For this review, take the finished solid that the model builds, in its own axes (mm). A direction names the side the tool comes from. Coordinates: 2 decimals unless noted, no trailing zeros. Loops run counter-clockwise (first coordinate to the right, second up) from the corner with the lowest first, then second, coordinate; pieces in that order, holes last.
1. Machinability: for faces 5 (the face through (0, -2, -76)), 6 (the face through (-24.577, 1.657, -55.458)), 7 (the face through (-74, -2, 10)), 8 (the face through (1.156, 0.908, -76.264)), 9 (the face through (8.684, -1.972, 16.654)), which of the approach directions +Z, -Z, +X, -X, +Y, -Y give a long, thin tool a straight path to every point of the face, cutting with its end or side? Answer none if there is none.
2. Take a section at B-B, the plane z = -50. State the section outline as (x, y) points, then the cut area to 3 significant figures.
3. Clearance check with flat-ended pins moving along their axes: P1, Ø2.5, axis at x = -8.75, z = -15.16, coming from the +Y side; P2, Ø5, axis at x = -8.75, z = 15.16, coming from the +Y side; P3, Ø3, axis at x = -43.5, z = -1.5, coming from the +Y side; P4, Ø8, axis at y = 5.5, z = -23.5, coming from the +X side. State where each tip first meets the part, or that it passes through.
4. Mouldability with a two-part tool opening along Y and no side actions: class faces 1 (the face through (76.066, 0.908, -3.422)), 2 (the face through (-1, -2, 26)), 3 (the face through (1, -4, -13)), 4 (the face through (27, 14.523, 18)) as pulls with the +Y half, pulls with the -Y half, needs draft (parallel to the pull), parting line crosses it, or undercut.
5. Take a section at A-A, the plane y = 9.5. State the section outline as (x, z) points, then the cut area to 3 significant figures.
6. To check wall thickness, follow probe 1 along X at (y, z) = (-1.25, -16); probe 2 along Z at (x, y) = (-46, 8.25); probe 3 along Z at (x, y) = (6, 10.75). State the ranges of each line that lie inside material, in increasing order.
```python
from build123d import *

# Parameters (mm, degrees)
SKETCH_1_R          = 26
EXTRUDE_1_DEPTH     = 1
EXTRUDE_1_2_DEPTH   = 1
EXTRUDE_1_3_DEPTH   = 1
EXTRUDE_START       = 4
SKETCH_2_R          = 10
EXTRUDE_2_DEPTH     = 4
SKETCH_3_R          = 1.5
CUT_EXTRUDE_1_DEPTH = 4


with BuildPart() as part:
    # Sketch 1 → Extrude 1 (new body)
    with BuildSketch(Plane(origin=(0, 0, 0), x_dir=(1, 0, 0), z_dir=(0, 1, 0))):
        with Locations(Location((0, 50, 0), (0, 0, 270))):
            Circle(SKETCH_1_R)
    extrude(amount=EXTRUDE_1_DEPTH)



with BuildPart() as body_2:
    # Sketch 1 → Extrude 1 2 (new body)
    with BuildSketch(Plane(origin=(0, 0, 0), x_dir=(1, 0, 0), z_dir=(0, 1, 0))):
        with Locations(Location((50, 0, 0), (0, 0, 270))):
            Circle(SKETCH_1_R)
    extrude(amount=EXTRUDE_1_2_DEPTH)


with BuildPart() as body_3:
    # Sketch 1 → Extrude 1 3 (new body)
    with BuildSketch(Plane(origin=(0, 0, 0), x_dir=(1, 0, 0), z_dir=(0, 1, 0))):
        with Locations(Location((-50, 0, 0), (0, 0, 270))):
            Circle(SKETCH_1_R)
    extrude(amount=EXTRUDE_1_3_DEPTH)


with BuildPart() as part_1:
    add(part.part)

    add(body_2.part)  # Extrude 2 merges body 2

    add(body_3.part)  # Extrude 2 merges body 3
    # Sketch 2 → Extrude 2 (add)
    with BuildSketch(Plane.XZ.offset(EXTRUDE_START)):
        with BuildLine():
            Line((-50, 26), (50, 26))
            ThreePointArc((50, 26), (74.020867845, 9.949769241), (68.384776311, -18.384776311))
            Line((68.384776311, -18.384776311), (18.384776311, -68.384776311))
            ThreePointArc((18.384776311, -68.384776311), (0, -76), (-18.384776311, -68.384776311))
            Line((-18.384776311, -68.384776311), (-68.384776311, -18.384776311))
            ThreePointArc((-68.384776311, -18.384776311), (-74.020867845, 9.949769241), (-50, 26))
        make_face()
        with Locations(Location((0, 0, 0), (0, 0, 270))):
            Circle(SKETCH_2_R, mode=Mode.SUBTRACT)
    extrude(amount=-EXTRUDE_2_DEPTH)

    # Sketch 3 → Cut-Extrude 1 (cut)
    with BuildSketch(Plane(origin=(0, 0, 0), x_dir=(1, 0, 0), z_dir=(0, 1, 0))):
        with Locations(Location((8.75, 15.155444566, 0), (0, 0, 270))):
            Circle(SKETCH_3_R)
        with Locations(Location((17.5, 0, 0), (0, 0, 270))):
            Circle(SKETCH_3_R)
        with Locations(Location((-17.5, 0, 0), (0, 0, 90))):
            Circle(SKETCH_3_R)
        with Locations(Location((-8.75, 15.155444566, 0), (0, 0, 90))):
            Circle(SKETCH_3_R)
        with Locations(Location((-8.75, -15.155444566, 0), (0, 0, 270))):
            Circle(SKETCH_3_R)
        with Locations(Location((8.75, -15.155444566, 0), (0, 0, 90))):
            Circle(SKETCH_3_R)
    extrude(amount=-CUT_EXTRUDE_1_DEPTH, mode=Mode.SUBTRACT)

    # Sketch 4 → Revolve 1 (revolve)
    with BuildSketch(Plane(origin=(0, 0, 0), x_dir=(0, 0, -1), z_dir=(1, 0, 0)), mode=Mode.PRIVATE) as revolve_1_sk:
        Polygon((80.623466631, 14.522961568), (78.623466631, 14.522961568), (75, 1), (76, 1), (76, 0), align=None)
    revolve(revolve_1_sk.sketch.rotate(Axis((0, 1, -50), (0, 1, 0)), 180), axis=Axis((0, 1, -50), (0, 1, 0)))

    # Sketch 6 → Revolve 2 (revolve)
    with BuildSketch(Plane.XY, mode=Mode.PRIVATE) as revolve_2_sk:
        Polygon((-75, 1), (-78.623466631, 14.522961568), (-80.623466631, 14.522961568), (-76, 0), (-76, 1), align=None)
    revolve(revolve_2_sk.sketch.rotate(Axis((-50, 1, 0), (0, 1, 0)), 90), axis=Axis((-50, 1, 0), (0, 1, 0)))

    # Sketch 7 → Revolve 3 (revolve)
    with BuildSketch(Plane.XY, mode=Mode.PRIVATE) as revolve_3_sk:
        Polygon((75, 1), (76, 1), (76, 0), (80.623466631, 14.522961568), (78.623466631, 14.522961568), align=None)
    revolve(revolve_3_sk.sketch.rotate(Axis((50, 1, 0), (0, 1, 0)), 270), axis=Axis((50, 1, 0), (0, 1, 0)))


solid = part_1.part
```
Results list:
1. face 5: -Z, -Y
1. face 6: +Y
1. face 7: -X, -Y
1. face 8: none
1. face 9: +Y, -Y
2. outline: (-36.77, -4) - (36.77, -4) - (36.77, 0) - (26, 0) - (30.62, 14.52) - (28.62, 14.52) - (25, 1) - (-25, 1) - (-28.62, 14.52) - (-30.62, 14.52) - (-26, 0) - (-36.77, 0) - close
2. area: 391 mm2
3. P1: passes through
3. P2: stops at y = 0
3. P3: stops at y = 1
3. P4: stops at x = 70.13
4. face 1: undercut
4. face 2: needs draft
4. face 3: pulls with the -Y half
4. face 4: pulls with the +Y half
5. outline: circle Ø58.05 at (-50, 0); circle Ø58.05 at (0, -50); circle Ø58.05 at (50, 0); hole circle Ø54.56 at (-50, 0); hole circle Ø54.56 at (0, -50); hole circle Ø54.56 at (50, 0)
5. area: 927 mm2
6. probe 1: x = -70.49 to -9.99, -7.51 to 7.51, 9.99 to 70.49
6. probe 2: z = -28.35 to -26.64, 26.64 to 28.35
6. probe 3: z = -78.8 to -76.95, -23.05 to -21.2
